Here's how the part is built. I have some questions about the finished solid (model axes, mm). Face numbers are marked on the shaded views. Coordinates: 2 decimals unless noted, no trailing zeros. Order: outer loops, then holes, each group sorted by start corner. A loop starts at its lowest first (then second) coordinate and runs counter-clockwise, first axis right, second up. Notation, with made-up numbers: (2.25, 5) - (60.25, 5) arc R35 cw to (60.25, 37) - close; hole circle Ø3 at (18, 41.5). An arc over 180 degrees is marked (long way). Answer in a Markdown table with one row per item. Add a question column.
Item 1: If I drill on line 1 along X through (y, z) = (26.5, 56); line 2 along Z through (x, y) = (68, 21.5); line 3 along Y through (x, z) = (-29.5, 52.5), over which ranges is the centre line in solid material (lowest first)? Write a range as from..to.
Item 2: I want a section at B-B (z = 50.5). Please give me the cut outline in (x, y).
Item 3: I want a section at C-C (z = -4). Please give me the cut outline in (x, y).
Item 4: Will these pins go through, and if not, where does the flat tip stop? pin 1 Ø10 at (x, z) = (7.5, -6) entering from +Y; pin 2 Ø10 at (x, z) = (19, 28) entering from -Y; pin 3 Ø3 at (x, z) = (-43.5, 47.5) entering from +Y; pin 4 Ø4.5 at (x, z) = (2.5, 17) entering from +Y.
Item 5: I want a section at A-A (x = 15). Please give me the cut outline in (y, z), plus the area to 3 significant figures.
Item 6: Thinking about a two-plate mould opening in Y: for the marked faces 1, 2 and 3, which applies, +Y half, -Y half, draft (parallel to the pull), parting line (faces both ways), or undercut?
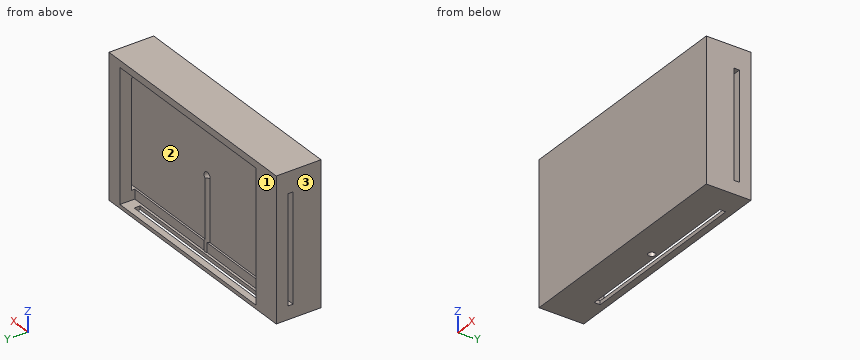
```python
from build123d import *

# Parameters (mm, degrees)
SKETCH1_W               = 160
SKETCH1_H               = 95
BOSS_EXTRUDE1_DEPTH     = 30
SKETCH3_W               = 130
SKETCH3_H               = 88
CUT_EXTRUDE1_DEPTH      = 10
SKETCH4_W               = 120.10834505
SKETCH4_H               = 4.01773352
CUT_EXTRUDE2_DEPTH      = 5
CUT_EXTRUDE4_START      = 10
SKETCH6_W               = 72.05939184
SKETCH6_H               = 3.5
CUT_EXTRUDE4_DEPTH      = 1
CUT_EXTRUDE4_DEPTH_BACK = 171
SKETCH7_R               = 2.3
CUT_EXTRUDE5_DEPTH      = 50
SKETCH8_R               = 2.907178759
CUT_EXTRUDE6_DEPTH      = 5


with BuildPart() as part:
    # Sketch1 → Boss-Extrude1 (new body)
    with BuildSketch(Plane(origin=(0, 0, 0), x_dir=(1, 0, 0), z_dir=(0, 1, 0))):
        with Locations((-0.236733524, -14.477499078)):
            Rectangle(SKETCH1_W, SKETCH1_H)
    extrude(amount=BOSS_EXTRUDE1_DEPTH)

    # Sketch3 → Cut-Extrude1 (cut)
    with BuildSketch(Plane(origin=(0, 30, 0), x_dir=(1, 0, 0), z_dir=(0, 1, 0))):
        with Locations((4.347428577, -13.440922118)):
            Rectangle(SKETCH3_W, SKETCH3_H)
    extrude(amount=-CUT_EXTRUDE1_DEPTH, mode=Mode.SUBTRACT)

    # Sketch4 → Cut-Extrude2 (cut)
    with BuildSketch(Plane(origin=(0, 0, -33.022500922), x_dir=(-1, 0, 0), z_dir=(0, 0, -1))):
        with Locations((-1.719856556, 23.682368484)):
            Rectangle(SKETCH4_W, SKETCH4_H)
    extrude(amount=-CUT_EXTRUDE2_DEPTH, mode=Mode.SUBTRACT)

    # Sketch6 → Cut-Extrude4 (cut, two sides)
    with BuildSketch(Plane(origin=(79.763266476, 0, 0), x_dir=(0, 0, -1), z_dir=(1, 0, 0)).offset(CUT_EXTRUDE4_START)) as cut_extrude4_sk:
        with Locations((-11.823423429, 20.472568853)):
            Rectangle(SKETCH6_W, SKETCH6_H)
    extrude(amount=CUT_EXTRUDE4_DEPTH, mode=Mode.SUBTRACT)
    extrude(cut_extrude4_sk.sketch, amount=-CUT_EXTRUDE4_DEPTH_BACK, mode=Mode.SUBTRACT)

    # Sketch7 → Cut-Extrude5 (cut)
    with BuildSketch(Plane(origin=(-65.187547899, 5.789113432, -33.022500922), x_dir=(-1, 0, 0), z_dir=(0, 0, -1))):
        with Locations((-66.824710363, 12.43513753)):
            Circle(SKETCH7_R)
    extrude(amount=-CUT_EXTRUDE5_DEPTH, mode=Mode.SUBTRACT)

    # Sketch8 → Cut-Extrude6 (cut)
    with BuildSketch(Plane(origin=(0, 20, 0), x_dir=(1, 0, 0), z_dir=(0, 1, 0))):
        with Locations((1.966492652, -16.875229275)):
            Circle(SKETCH8_R)
    extrude(amount=-CUT_EXTRUDE6_DEPTH, mode=Mode.SUBTRACT)


solid = part.part
```
Values follow:
| question | item | result |
|---|---|---|
| 1 | line 1 | x = -80.24..-60.65, 69.35..79.76 |
| 1 | line 2 | z = -33.02..-30.56, 57.44..61.98 |
| 1 | line 3 | y = 0..20 |
| 2 | outline | (-80.24, 0) - (79.76, 0) - (79.76, 30) - (69.35, 30) - (69.35, 20) - (-60.65, 20) - (-60.65, 30) - (-80.24, 30) - close |
| 3 | outline | (-80.24, 0) - (79.76, 0) - (79.76, 18.72) - (3.88, 18.72) arc R2.3 cw (long way) to (-0.61, 18.72) - (-80.24, 18.72) - close; (-80.24, 22.22) - (-60.65, 22.22) - (-60.65, 30) - (-80.24, 30) - close; (69.35, 22.22) - (79.76, 22.22) - (79.76, 30) - (69.35, 30) - close |
| 4 | pin 1 | stops at y = 18.72 |
| 4 | pin 2 | stops at y = 0 |
| 4 | pin 3 | stops at y = 20 |
| 4 | pin 4 | stops at y = 15 |
| 5 | outline | (0, -33.02) - (21.67, -33.02) - (21.67, -30.56) - (20, -30.56) - (20, -24.21) - (18.72, -24.21) - (18.72, 47.85) - (20, 47.85) - (20, 57.44) - (30, 57.44) - (30, 61.98) - (0, 61.98) - close; (25.69, -33.02) - (30, -33.02) - (30, -30.56) - (25.69, -30.56) - close |
| 5 | area | 1,870 mm^2 |
| 6 | face 1 | +Y half |
| 6 | face 2 | undercut |
| 6 | face 3 | draft |
